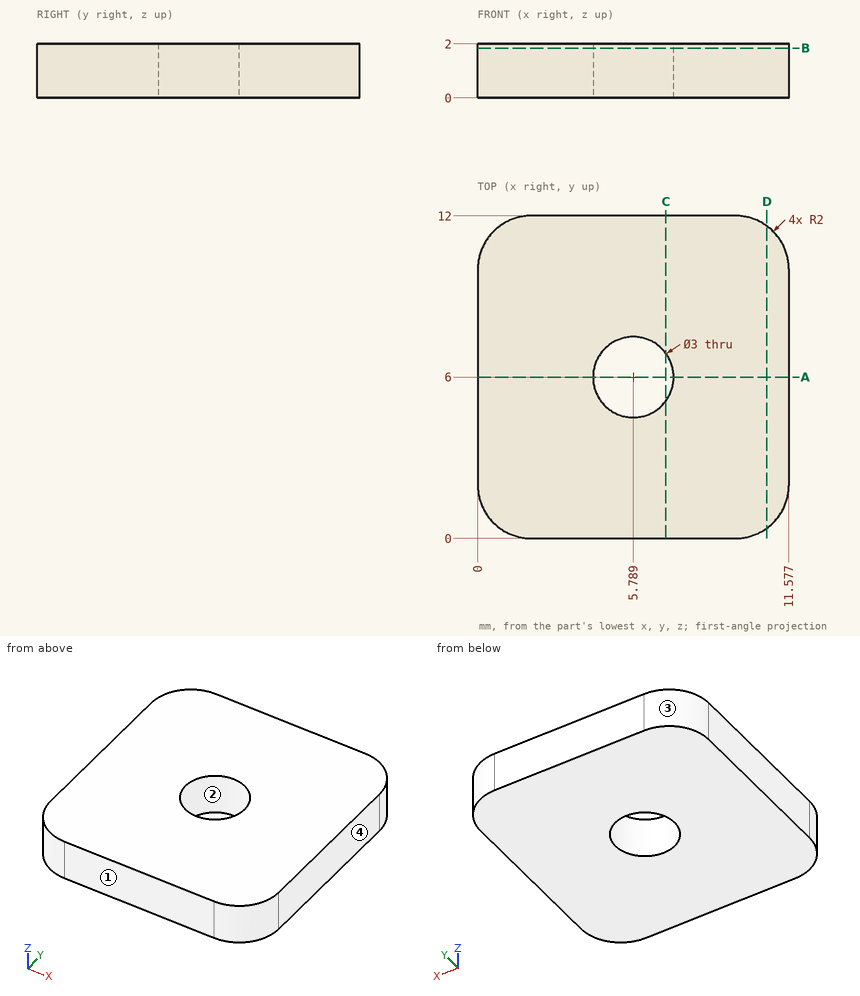
Can you work these out from the drawing? Everything is in mm from the part's minimum corner. Give positions to 0.01 mm unless a question says otherwise; leave off trailing zeros. Order: outer loops, then holes, each group sorted by start corner. A loop starts at its lowest first (then second) coordinate and runs counter-clockwise, first axis right, second up. Notation, with made-up numbers: M 61.5,21 L 105.5,21 A27 cw 105.5,50 Z; hole C 18.25,33 d11. An arc over 180 degrees is marked long. Write item = value, one per line. Start each with the question number.
Q1. Suppose I cut it at C-C (x = 7). Write out the boundary of the cut face in (y, z) (1 decimal).
Q2. Suppose I cut it at D-D (x = 10.75). Write out the boundary of the cut face in (y, z).
Q3. We'd pull the mould along X, two halves only. Please class the marked faces 1, 2, 3 and 4: pulls with the +X half, pulls with the -X half, needs draft (parallel to the pull), parting line crosses it, or undercut.
Q4. Will this pin go through, and if not, where does the flat tip stop? pin 1 Ø1.8 at (x, y) = (5.79, 6) entering from -Z.
Q5. Suppose I cut it at B-B (z = 1.85). Write out the boundary of the cut face in (x, y), plus the area to 3 significant figures.
Q6. Suppose I cut it at A-A (y = 6). Write out the boundary of the cut face in (x, z).
Q7. I need wall thicknesses on probe 1 along Y at (x, z) = (5.75, 0.4); probe 2 along X at (y, z) = (5.25, 1.3); probe 3 along X at (y, z) = (7.25, 0.8) (1 decimal). Which ranges of each line are inside material? Lowest first, please. Write a range as [from, to].
Check result:
q1.outline = M 0,0 L 5.1,0 L 5.1,2 L 0,2 Z; M 6.9,0 L 12,0 L 12,2 L 6.9,2 Z
q2.outline = M 0.38,0 L 11.62,0 L 11.62,2 L 0.38,2 Z
q3.face_1 = needs draft
q3.face_2 = undercut
q3.face_3 = pulls with the -X half
q3.face_4 = pulls with the +X half
q4.pin_1 = through
q5.outline = M 0,2 A2 ccw 2,0 L 9.58,0 A2 ccw 11.58,2 L 11.58,10 A2 ccw 9.58,12 L 2,12 A2 ccw 0,10 Z; hole C 5.79,6 d3
q5.area = 128 mm2
q6.outline = M 0,0 L 4.29,0 L 4.29,2 L 0,2 Z; M 7.29,0 L 11.58,0 L 11.58,2 L 7.29,2 Z
q7.probe_1 = [0, 4.5], [7.5, 12]
q7.probe_2 = [0, 4.49], [7.09, 11.58]
q7.probe_3 = [0, 5], [6.6, 11.6]
